Can you work these out from the model? Positions are in its coordinate system, mm. A direction names the side the tool comes from. Round coordinates to 2 decimals unless told otherwise and drop trailing zeros. Write each loop counter-clockwise with the first axis right and the second up, starting at its lowest first coordinate (ties: lowest second). Pieces come first, ordered by that corner, then holes. Notation, with made-up numbers: M -7.75,22 L 37.25,22 A27 ccw 37.25,59 Z; hole C 58.25,36 d7. An arc over 180 degrees is marked long. Answer as a JSON object with one key per item and string values. Group by question number.
1) I'm going to push flat-ended pins straight in: pin 1 Ø5 at (x, y) = (-3.5, -5) entering from -Z; pin 2 Ø1.1 at (x, z) = (4.5, 2) entering from -Y; pin 3 Ø1 at (x, y) = (-4.5, -6) entering from +Z. Where does each tip first touch, or does it pass through?
2) Suppose I cut it at C-C, the plane x = 5. Write out the boundary of the cut face in (y, z).
3) On a 3-axis mill with a long thin cutter (end or side, diameter ignored), from which of +Z, -Z, +X, -X, +Y, -Y can I reach the whole of each face in a straight line? I mean faces 1 (the cylindrical face through (-0.13, 4.946, -2.049)), 2 (the flat face through (0, 6, 1.1)), 3 (the flat face through (0, -4.95, 2)). Say none if no direction works.
4) Suppose I cut it at D-D, the plane y = -1.75. Write out the boundary of the cut face in (x, z).
5) Suppose I cut it at B-B, the plane x = 0. Write out the boundary of the cut face in (y, z).
6) Suppose I cut it at A-A, the plane y = 0. Write out the boundary of the cut face in (x, z).
7) Please list where these lines run through material, in increasing order: L1, parallel to Y at x = 0, z = 0.7; L2, parallel to Y at x = 0, z = -0.5; L3, parallel to Z at x = 2, y = -3. Write a range as [from, to].
from build123d import *

# Parameters (mm, degrees)
BOSS_EXTRUDE1_DEPTH      = 9.5
BOSS_EXTRUDE1_DEPTH_BACK = 9.5
SKETCH6_R                = 2.413
CUT_EXTRUDE2_DEPTH       = 13.895347998
FILLET5_R                = 0.25


with BuildPart() as part:
    # Sketch4 → Boss-Extrude1 (new, two sides: drawn at the far end of the back side and taken through both)
    with BuildSketch(Plane(origin=(0, 0, 0), x_dir=(0, 0, -1), z_dir=(1, 0, 0)).offset(-BOSS_EXTRUDE1_DEPTH_BACK)):
        with BuildLine():
            Line((-0.35, 6.933012702), (0.6, 6.384529946))
            ThreePointArc((0.6, 6.384529946), (2.064101615, 4.920428331), (2.6, 2.920428331))
            Line((2.6, 2.920428331), (2.6, -2.920428331))
            ThreePointArc((2.6, -2.920428331), (2.064101615, -4.920428331), (0.6, -6.384529946))
            Line((0.6, -6.384529946), (-0.35, -6.933012702))
            ThreePointArc((-0.35, -6.933012702), (-0.85, -6.933012702), (-1.1, -6.5))
            Line((-1.1, -6.5), (-1.1, -4.95))
            Line((-1.1, -4.95), (-2.6, -4.95))
            Line((-2.6, -4.95), (-2.6, 4.95))
            Line((-2.6, 4.95), (-1.1, 4.95))
            Line((-1.1, 4.95), (-1.1, 6.5))
            ThreePointArc((-1.1, 6.5), (-0.85, 6.933012702), (-0.35, 6.933012702))
        make_face()
    extrude(amount=BOSS_EXTRUDE1_DEPTH + BOSS_EXTRUDE1_DEPTH_BACK)

    # Sketch6 → Cut-Extrude2 (cut, through all)
    with BuildSketch(Plane.XY.offset(2.6)):
        Circle(SKETCH6_R)
    extrude(amount=-CUT_EXTRUDE2_DEPTH, mode=Mode.SUBTRACT)

    # Fillet5
    fillet5_edges = [part.edges().sort_by_distance(p)[0] for p in [
        (-9.5, 4.920428331, -2.064101615),
        (-9.5, 6.658771324, -0.125),
        (-9.5, 6.933012702, 0.85),
        (-9.5, 5.725, 1.1),
        (0, -4.95, 1.1),
        (0, -4.95, 2.6),
        (0, 4.95, 2.6),
        (0, 4.95, 1.1),
        (-9.5, 4.95, 1.85),
        (-9.5, 0, 2.6),
        (-9.5, -4.95, 1.85),
        (-9.5, -5.725, 1.1),
        (9.5, -4.920428331, -2.064101615),
        (9.5, 0, -2.6),
        (9.5, 4.920428331, -2.064101615),
        (-9.5, -6.933012702, 0.85),
        (9.5, 6.658771324, -0.125),
        (9.5, 6.933012702, 0.85),
        (9.5, 5.725, 1.1),
        (9.5, 4.95, 1.85),
        (9.5, 0, 2.6),
        (9.5, -4.95, 1.85),
        (9.5, -5.725, 1.1),
        (9.5, -6.933012702, 0.85),
        (9.5, -6.658771324, -0.125),
        (-9.5, -6.658771324, -0.125),
        (-9.5, -4.920428331, -2.064101615),
        (-9.5, 0, -2.6),
    ]]
    fillet(fillet5_edges, radius=FILLET5_R)


solid = part.part
Results:
{
 "1": {"pin 1": "z = -2.6", "pin 2": "y = -4.95", "pin 3": "z = 1.1"},
 "2": {"outline": "M -6.93,0.35 L -6.38,-0.6 A4 ccw -2.92,-2.6 L 2.92,-2.6 A4 ccw 6.38,-0.6 L 6.93,0.35 A0.5 ccw 6.5,1.1 L 5.2,1.1 A0.25 cw 4.95,1.35 L 4.95,2.35 A0.25 ccw 4.7,2.6 L -4.7,2.6 A0.25 ccw -4.95,2.35 L -4.95,1.35 A0.25 cw -5.2,1.1 L -6.5,1.1 A0.5 ccw Z"},
 "3": {"face 1": "-Z, +X, -X, +Y", "face 2": "+Z, +X, -X, +Y", "face 3": "+Z, +X, -X, -Y"},
 "4": {"outline": "M -9.5,-2.35 A0.25 ccw -9.25,-2.6 L -1.66,-2.6 L -1.66,2.6 L -9.25,2.6 A0.25 ccw -9.5,2.35 Z; M 1.66,-2.6 L 9.25,-2.6 A0.25 ccw 9.5,-2.35 L 9.5,2.35 A0.25 ccw 9.25,2.6 L 1.66,2.6 Z"},
 "5": {"outline": "M -6.93,0.35 L -6.38,-0.6 A4 ccw -2.92,-2.6 L -2.41,-2.6 L -2.41,2.6 L -4.7,2.6 A0.25 ccw -4.95,2.35 L -4.95,1.35 A0.25 cw -5.2,1.1 L -6.5,1.1 A0.5 ccw Z; M 2.41,-2.6 L 2.92,-2.6 A4 ccw 6.38,-0.6 L 6.93,0.35 A0.5 ccw 6.5,1.1 L 5.2,1.1 A0.25 cw 4.95,1.35 L 4.95,2.35 A0.25 ccw 4.7,2.6 L 2.41,2.6 Z"},
 "6": {"outline": "M -9.5,-2.35 A0.25 ccw -9.25,-2.6 L -2.41,-2.6 L -2.41,2.6 L -9.25,2.6 A0.25 ccw -9.5,2.35 Z; M 2.41,-2.6 L 9.25,-2.6 A0.25 ccw 9.5,-2.35 L 9.5,2.35 A0.25 ccw 9.25,2.6 L 2.41,2.6 Z"},
 "7": {"L1": "[-6.99, -2.41], [2.41, 6.99]", "L2": "[-6.44, -2.41], [2.41, 6.44]", "L3": "[-2.6, 2.6]"}
}
